from build123d import *

# Parameters (mm, degrees)
F1_DEPTH = 92
F2_W     = 19.621109
F2_H     = 76
F2_W_2   = 27.378891
F3_DEPTH = 10


with BuildPart() as f1:
    # F0 (on Top) → F1 (new body)
    with BuildSketch(Plane.XY):
        Polygon((-46, 45.39616), (-46, -46.60384), (-29.854571, -46.60384), (0, 22.311091), (29.854571, -46.60384), (46, -46.60384), (46, 45.39616), (32, 45.39616), (32, -16.067849), (5.373236, 45.39616), (0, 45.39616), (-5.373236, 45.39616), (-32, -16.067849), (-32, 45.39616), align=None)
    extrude(amount=-F1_DEPTH)

    # F2 (on face) → F3 (cut)
    with BuildSketch(Plane.YZ.offset(46)):
        with Locations((20.585605, -53)):
            Rectangle(F2_W, F2_H)
        with Locations((-17.914395, -39)):
            Rectangle(F2_W_2, F2_H)
    extrude(amount=-F3_DEPTH, mode=Mode.SUBTRACT)


solid = f1.part
Geometry check sheet. Reference: the model listing, model coordinates, mm. A direction names the side the tool comes from. Coordinates: 2 decimals unless noted, no trailing zeros. Loops run counter-clockwise (first coordinate to the right, second up) from the corner with the lowest first, then second, coordinate; pieces in that order, holes last. Notation, with made-up numbers: (-40, 70.25) - (-3, 70.25) arc R32 ccw to (-3, 109.25) - close; hole circle Ø3 at (23.5, 3). An arc over 180 degrees is marked (long way). Use one line per item in the form item = value. Start each with the question number.
Item 1: Tool access check on faces 1 (the face through (41, -18, -77)), 2 (the face through (39, 45.396, -45)), 3 (the face through (18.873, 14.234, -45.356)). Record the directions out of +Z, -Z, +X, -X, +Y, -Y that give a thin tool (end or side, any length) a straight path to the whole face; none if there is none.
Item 2: Section check B-B, the plane z = -41. Enter the section's corners in (x, y), and give its area (3 significant figures).
Item 3: Section check D-D, the plane y = 25.5. Enter the section's corners in (x, z), and give its area (3 significant figures).
Item 4: Section check C-C, the plane y = -6.5. Enter the section's corners in (x, z), and give its area (3 significant figures).
Item 5: Mould release check, pull along X, two halves, no side actions. Record for faces 4 (the face through (14.718, -11.664, -45.356)), 5 (the face through (41, 10.775, -54)), 6 (the face through (46, -1, -45)): +X half, -X half, draft (parallel to the pull), parting line (faces both ways), or undercut.
Item 6: Section check A-A, the plane y = -27. Enter the section's corners in (x, z).
Item 7: Gauge pin test, flat ends, axial feed: pin 1 (22 mm diameter, centred on y = -19, z = -23.5, fed in from +X); pin 2 (1 mm diameter, centred on x = 28, z = -33.5, fed in from +Y); pin 3 (2 mm diameter, centred on x = 16.5, z = -43, fed in from +Y). Record the tip position at first contact, or that the pin passes through.
Item 8: Thickness scan on probe 1 along Y at (x, z) = (39.5, -66); probe 2 along X at (y, z) = (-13, -19.5); probe 3 along X at (y, z) = (37.5, -64). Record the ranges inside material, lowest first.
Computed:
q1.face_1 = +X
q1.face_2 = +Z, -Z, +X, -X, +Y
q1.face_3 = +Z, -Z, +Y
q2.outline = (-46, -46.6) - (-29.85, -46.6) - (0, 22.31) - (29.85, -46.6) - (46, -46.6) - (46, -31.6) - (36, -31.6) - (36, -4.22) - (46, -4.22) - (46, 10.78) - (36, 10.78) - (36, 30.4) - (46, 30.4) - (46, 45.4) - (32, 45.4) - (32, -16.07) - (5.37, 45.4) - (-5.37, 45.4) - (-32, -16.07) - (-32, 45.4) - (-46, 45.4) - close
q2.area = 4,300 mm2
q3.outline = (-46, -92) - (-32, -92) - (-32, 0) - (-46, 0) - close; (-13.99, -92) - (13.99, -92) - (13.99, 0) - (-13.99, 0) - close; (32, -92) - (46, -92) - (46, -91) - (36, -91) - (36, -15) - (46, -15) - (46, 0) - (32, 0) - close
q3.area = 4,390 mm2
q4.outline = (-46, -92) - (-32, -92) - (-32, 0) - (-46, 0) - close; (-27.86, -92) - (-12.48, -92) - (-12.48, 0) - (-27.86, 0) - close; (12.48, -92) - (27.86, -92) - (27.86, 0) - (12.48, 0) - close; (32, -92) - (46, -92) - (46, -77) - (36, -77) - (36, -1) - (46, -1) - (46, 0) - (32, 0) - close
q4.area = 4,640 mm2
q5.face_4 = undercut
q5.face_5 = draft
q5.face_6 = +X half
q6.outline = (-46, -92) - (-21.36, -92) - (-21.36, 0) - (-46, 0) - close; (21.36, -92) - (46, -92) - (46, -77) - (36, -77) - (36, -1) - (46, -1) - (46, 0) - (21.36, 0) - close
q7.pin_1 = 36
q7.pin_2 = -5.68
q7.pin_3 = 22.02
q8.probe_1 = -46.6 to -31.6, -4.22 to 10.78, 30.4 to 45.4
q8.probe_2 = -46 to -32, -30.67 to -15.3, 15.3 to 30.67, 32 to 36
q8.probe_3 = -46 to -32, -8.79 to 8.79, 32 to 46
